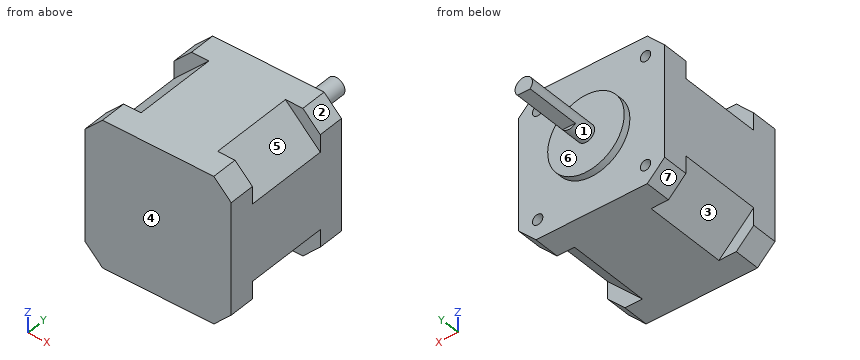
from build123d import *

# Parameters (mm, degrees)
EXTRUDE_1_DEPTH     = 7.5
EXTRUDE_2_DEPTH     = 24
EXTRUDE_3_DEPTH     = 7.5
SKETCH_4_R          = 11
EXTRUDE_4_DEPTH     = 2
SKETCH_5_R          = 2.5
EXTRUDE_5_DEPTH     = 22
SKETCH_6_W          = 7.205665958
SKETCH_6_H          = 1.954366946
CUT_EXTRUDE_1_DEPTH = 16
SKETCH_7_R          = 1.5
CUT_EXTRUDE_2_DEPTH = 5


with BuildPart() as part:
    # 草图1 → 凸台-拉伸1 (new body)
    with BuildSketch(Plane(origin=(0, 0, 0), x_dir=(1, 0, 0), z_dir=(0, 1, 0))):
        Polygon((-21, 16), (-16, 21), (16, 21), (21, 16), (21, -16), (16, -21), (-16, -21), (-21, -16), align=None)
    extrude(amount=-EXTRUDE_1_DEPTH)

    # 草图2 → 凸台-拉伸2 (add)
    with BuildSketch(Plane.XZ.offset(7.5)):
        Polygon((-21, 11), (-11, 21), (11, 21), (21, 11), (21, -11), (11, -21), (-11, -21), (-21, -11), align=None)
    extrude(amount=EXTRUDE_2_DEPTH)

    # 草图3 → 凸台-拉伸3 (add)
    with BuildSketch(Plane.XZ.offset(31.5)):
        Polygon((-21, 16), (-16, 21), (16, 21), (21, 16), (21, -16), (16, -21), (-16, -21), (-21, -16), align=None)
    extrude(amount=EXTRUDE_3_DEPTH)

    # 草图4 → 凸台-拉伸4 (add)
    with BuildSketch(Plane(origin=(0, 0, 0), x_dir=(1, 0, 0), z_dir=(0, 1, 0))):
        with Locations(Location((0, 0, 0), (0, 0, 270))):
            Circle(SKETCH_4_R)
    extrude(amount=EXTRUDE_4_DEPTH)

    # 草图5 → 凸台-拉伸5 (add)
    with BuildSketch(Plane(origin=(0, 2, 0), x_dir=(1, 0, 0), z_dir=(0, 1, 0))):
        with Locations(Location((0, 0, 0), (0, 0, 270))):
            Circle(SKETCH_5_R)
    extrude(amount=EXTRUDE_5_DEPTH)

    # 草图6 → 切除-拉伸1 (cut)
    with BuildSketch(Plane(origin=(0, 24, 0), x_dir=(1, 0, 0), z_dir=(0, 1, 0))):
        with Locations((0.108418899, 2.670655674)):
            Rectangle(SKETCH_6_W, SKETCH_6_H)
    extrude(amount=-CUT_EXTRUDE_1_DEPTH, mode=Mode.SUBTRACT)

    # 草图7 → 切除-拉伸2 (cut)
    with BuildSketch(Plane(origin=(0, 0, 0), x_dir=(1, 0, 0), z_dir=(0, 1, 0))):
        with Locations(Location((-15.5, 15.5, 0), (0, 0, 270))):
            Circle(SKETCH_7_R)
        with Locations(Location((15.5, 15.5, 0), (0, 0, 270))):
            Circle(SKETCH_7_R)
        with Locations(Location((15.5, -15.5, 0), (0, 0, 270))):
            Circle(SKETCH_7_R)
        with Locations(Location((-15.5, -15.5, 0), (0, 0, 270))):
            Circle(SKETCH_7_R)
    extrude(amount=-CUT_EXTRUDE_2_DEPTH, mode=Mode.SUBTRACT)


solid = part.part
Check sheet for the modelled part. Datum: model origin and axes. Units: mm. Face numbers are marked on the shaded views. A direction names the side the tool comes from. Round coordinates to 2 decimals unless told otherwise and drop trailing zeros. Loops run counter-clockwise (first coordinate to the right, second up) from the corner with the lowest first, then second, coordinate; pieces in that order, holes last. Notation, with made-up numbers: M 48.25,45.25 L 76.25,45.25 A11 ccw 76.25,63.25 Z; hole C -22.75,10 d4. An arc over 180 degrees is marked long. One line per question, with ' | ' between items. Start each with the question number.
Item 1: Section check D-D (z = -5.5). Record the boundary of the cut face in (x, y).
Item 2: Set-up check for the marked faces 1, 2 and 3: record each of +Z, -Z, +X, -X, +Y, -Y from which the full face is reachable in a straight line by a thin tool's end or side.
Item 3: Scan lines: probe 1 along Y at (x, z) = (15.5, -18); probe 2 along Z at (x, y) = (15, -2); probe 3 along Y at (x, z) = (13, -7). Record each from-to range of solid material in increasing order.
Item 4: Section check A-A (x = 0). Record the boundary of the cut face in (y, z).
Item 5: Gauge pin test, flat ends, axial feed: pin 1 Ø5 at (x, z) = (-15, -16.5) entering from +Y; pin 2 Ø1.8 at (x, y) = (0, 18) entering from -Z; pin 3 Ø6 at (x, y) = (-14.5, -25.5) entering from +Z. Record the tip position at first contact, or that the pin passes through.
Item 6: Section check B-B (z = 0). Record the boundary of the cut face in (x, y).
Item 7: Release check for a two-part mould opening along Y. For the marked faces 4, 5, 6 and 7 record: released by +Y, released by -Y, zero draft, split by the parting line, or undercut.
Item 8: Section check C-C (y = -25.5). Record the boundary of the cut face in (x, z).
Worked out:
1) outline: M -21,-39 L 21,-39 L 21,0 L 9.53,0 L 9.53,2 L -9.53,2 L -9.53,0 L -21,0 Z
2) face 1: +Y | face 2: +Z, +X, +Y, -Y | face 3: -Z, -X
3) probe 1: -39 to -31.5, -7.5 to 0 | probe 2: -21 to -16.91, -14.09 to 14.09, 16.91 to 21 | probe 3: -39 to 0
4) outline: M -39,-21 L 0,-21 L 0,-11 L 2,-11 L 2,-2.5 L 8,-2.5 L 8,-1.69 L 24,-1.69 L 24,2.5 L 2,2.5 L 2,11 L 0,11 L 0,21 L -39,21 Z
5) pin 1: y = 0 | pin 2: z = -1.69 | pin 3: z = 20.5
6) outline: M -21,-39 L 21,-39 L 21,0 L 11,0 L 11,2 L 2.5,2 L 2.5,24 L -2.5,24 L -2.5,2 L -11,2 L -11,0 L -21,0 Z
7) face 4: released by -Y | face 5: undercut | face 6: released by +Y | face 7: zero draft
8) outline: M -21,-11 L -11,-21 L 11,-21 L 21,-11 L 21,11 L 11,21 L -11,21 L -21,11 Z
